```python
from build123d import *

# Parameters (mm, degrees)
BOSS_EXTRUDE1_DEPTH                                 = 16
CSK_FOR_M3_COUNTERSUNK_FLAT_HEAD_SCREW1_D           = 3.4
CSK_FOR_M3_COUNTERSUNK_FLAT_HEAD_SCREW1_CSINK_D     = 6.3
CSK_FOR_M3_COUNTERSUNK_FLAT_HEAD_SCREW1_CSINK_ANGLE = 90
CUT_EXTRUDE1_DEPTH                                  = 9
SKETCH5_R                                           = 4.1
CUT_EXTRUDE2_DEPTH                                  = 6
SKETCH6_R                                           = 1.55
CUT_EXTRUDE3_DEPTH                                  = 106.750886521
SKETCH7_R                                           = 7
CUT_EXTRUDE4_DEPTH                                  = 2
FILLET1_R                                           = 8


with BuildPart() as part:
    # Sketch1 → Boss-Extrude1 (new body)
    with BuildSketch(Plane(origin=(0, 0, 0), x_dir=(0, 0, -1), z_dir=(1, 0, 0))):
        Polygon((0, 0), (-98.5, 0), (-98.5, 35), (5, 35), (5, 30), (0, 30), align=None)
    extrude(amount=BOSS_EXTRUDE1_DEPTH)

    # CSK for M3 Countersunk Flat Head Screw1 (through all)
    with Locations(Plane(origin=(16, 26, 88.5), x_dir=(0, 0, 1), z_dir=(1, 0, 0))):
        with Locations((0, 0), (0, 10), (-20, -4), (-20, 21), (-80, 0), (-80, 10)):
            CounterSinkHole(CSK_FOR_M3_COUNTERSUNK_FLAT_HEAD_SCREW1_D / 2, CSK_FOR_M3_COUNTERSUNK_FLAT_HEAD_SCREW1_CSINK_D / 2, counter_sink_angle=CSK_FOR_M3_COUNTERSUNK_FLAT_HEAD_SCREW1_CSINK_ANGLE)

    # Sketch4 → Cut-Extrude1 (cut)
    with BuildSketch(Plane.ZY):
        Polygon((10.0875, 28.749630657), (6.9125, 28.749630657), (5.325, 26), (6.9125, 23.250369343), (10.0875, 23.250369343), (11.675, 26), align=None)
        Polygon((86.9125, 28.749630657), (85.325, 26), (86.9125, 23.250369343), (90.0875, 23.250369343), (91.675, 26), (90.0875, 28.749630657), align=None)
    extrude(amount=-CUT_EXTRUDE1_DEPTH, mode=Mode.SUBTRACT)

    # Sketch5 → Cut-Extrude2 (cut)
    with BuildSketch(Plane.ZY):
        with Locations((8.5, 26)):
            Circle(SKETCH5_R)
        with Locations((88.5, 26)):
            Circle(SKETCH5_R)
    extrude(amount=-CUT_EXTRUDE2_DEPTH, mode=Mode.SUBTRACT)

    # Sketch6 → Cut-Extrude3 (cut, through all)
    with BuildSketch(Plane(origin=(16, 0, 0), x_dir=(0, 0, -1), z_dir=(1, 0, 0))):
        with Locations((-24, 13)):
            Circle(SKETCH6_R)
    extrude(amount=-CUT_EXTRUDE3_DEPTH, mode=Mode.SUBTRACT)

    # Sketch7 → Cut-Extrude4 (cut)
    with BuildSketch(Plane(origin=(16, 0, 0), x_dir=(0, 0, -1), z_dir=(1, 0, 0))):
        with Locations((-24, 13)):
            Circle(SKETCH7_R)
    extrude(amount=-CUT_EXTRUDE4_DEPTH, mode=Mode.SUBTRACT)

    # Fillet1
    fillet1_edges = [part.edges().sort_by_distance(p)[0] for p in [
        (8, 35, 98.5),
    ]]
    fillet(fillet1_edges, radius=FILLET1_R)


solid = part.part
```
Input: part model. Units: mm. Frame: model coordinates. A direction names the side the tool comes from. Coordinates: 2 decimals unless noted, no trailing zeros. Write each loop counter-clockwise with the first axis right and the second up, starting at its lowest first coordinate (ties: lowest second). Pieces come first, ordered by that corner, then holes. Notation, with made-up numbers: (24.5, -1) -> (62.5, -1) arc R31 ccw to (62.5, 37) -> close; hole circle Ø5 at (-14, -25.75). An arc over 180 degrees is marked (long way). Answer as a JSON object with one key per item and string values.
1. First-contact query: P1, Ø8.5, axis at y = 13, z = 24, coming from the -X side; P2, Ø1, axis at x = 3, y = 18.5, coming from the -Z side; P3, Ø11, axis at y = 14, z = 25, coming from the +X side; P4, Ø4, axis at y = 5, z = 68.5, coming from the +X side. Flat tips, straight axial feed; report the tip coordinate or a pass-through.
Result set:
{"P1": "stops at x = 0", "P2": "stops at z = 0", "P3": "stops at x = 14", "P4": "stops at x = 14.85"}
2. Section A-A on z = 68.5. Return the cut outline in (x, y).
Result set:
{"outline": "(0, 0) -> (16, 0) -> (16, 1.85) -> (14.55, 3.3) -> (0, 3.3) -> close; (0, 6.7) -> (14.55, 6.7) -> (16, 8.15) -> (16, 26.85) -> (14.55, 28.3) -> (0, 28.3) -> close; (0, 31.7) -> (14.55, 31.7) -> (16, 33.15) -> (16, 35) -> (0, 35) -> close"}
3. Section D-D on y = 10. Return the cut outline in (x, z), then the cut area to 3 significant figures.
Result set:
{"outline": "(0, 0) -> (16, 0) -> (16, 17.68) -> (14, 17.68) -> (14, 30.32) -> (16, 30.32) -> (16, 98.5) -> (0, 98.5) -> close", "area": "1,550 mm2"}
4. Material intervals for line 1 (Y direction, x = 8.25, z = 8.5); line 2 (Y direction, x = 3.95, z = 8.5); line 3 (Z direction, x = 8.5, y = 16), sorted ascending. Write a range as from..to.
Result set:
{"line 1": "y = 0..14.3, 17.7..23.25, 28.75..35", "line 2": "y = 0..14.3, 17.7..21.9, 30.1..35", "line 3": "z = 0..6.8, 10.2..86.8, 90.2..98.5"}
5. Access query for faces 1 (the face through (7.098, 12.406, 22.568)), 2 (the face through (2.958, 23.505, 5.246)), 3 (the face through (14, 13, 26)). Directions: +Z, -Z, +X, -X, +Y, -Y. A direction counts if a zero-diameter tool reaches every point of the face in a straight line with its end or side. Return the directions, or none.
Result set:
{"face 1": "+X, -X", "face 2": "-X", "face 3": "+X"}
6. Section C-C on y = 5. Return the cut outline in (x, z), then the cut area to 3 significant figures.
Result set:
{"outline": "(0, 0) -> (16, 0) -> (16, 65.35) -> (14.55, 66.8) -> (0, 66.8) -> close; (0, 70.2) -> (14.55, 70.2) -> (16, 71.65) -> (16, 98.5) -> (0, 98.5) -> close", "area": "1,520 mm2"}
7. Section B-B on z = 24. Return the cut outline in (x, y), then the cut area to 3 significant figures.
Result set:
{"outline": "(0, 0) -> (16, 0) -> (16, 6) -> (14, 6) -> (14, 11.45) -> (0, 11.45) -> close; (0, 14.55) -> (14, 14.55) -> (14, 20) -> (16, 20) -> (16, 35) -> (0, 35) -> close", "area": "489 mm2"}
8. Mould query, pull axis Y, two halves, no side actions, for faces 4 (the face through (8, 30, -3)), 5 (the face through (8, 35, 43)), 6 (the face through (9, 27.3, 9.9)). Classes: released by +Y, released by -Y, zero draft, split by the parting line, or undercut.
Result set:
{"face 4": "released by -Y", "face 5": "released by +Y", "face 6": "undercut"}
